from build123d import *

# Parameters (mm, degrees)
F3_START = -35.13478
F3_DEPTH = 29.12792
F4_SIZE  = 10.16
F5_R     = 93.5075941329
F6_DEPTH = 127


with BuildPart() as f1:
    # F0 (on Front) → F1 (revolve)
    with BuildSketch(Plane.XZ):
        Polygon((0, 127), (0, 0), (457.2, 0), (457.2, 38.1), (433.5165438938, 38.1), (433.5165438938, 106.68), (398.78, 106.68), (398.78, 152.4), (43.18, 152.4), (43.18, 127), align=None)
    revolve(axis=Axis((228.6, 0, 0), (1, 0, 0)))

    # F2 (on Top) → F3 (cut)
    with BuildSketch(Plane.XY.offset(F3_START)):
        with BuildLine():
            Line((435.6053211212, 11.4893475547), (390.5868865967, 11.4893475547))
            ThreePointArc((390.5868865967, 11.4893475547), (377.9254574746, -1.1720815673), (390.5868865967, -13.8335106894))
            Line((390.5868865967, -13.8335106894), (435.6053211212, -13.8335106894))
            ThreePointArc((435.6053211212, -13.8335106894), (448.2667502433, -1.1720815673), (435.6053211212, 11.4893475547))
        make_face()
    extrude(amount=-F3_DEPTH, mode=Mode.SUBTRACT)

    # F4
    f4_edges = [f1.edges().sort_by_distance(p)[0] for p in [
        (43.18, 0, -152.4),
        (398.78, 0, -152.4),
    ]]
    chamfer(f4_edges, length=F4_SIZE)

    # F5 (on face) → F6 (join)
    with BuildSketch(Plane(origin=(0, 0, 0), x_dir=(0, -1, 0), z_dir=(-1, 0, 0))):
        with Locations((-8.3505315706, -17.3037741333)):
            Circle(F5_R)
    extrude(amount=F6_DEPTH)


solid = f1.part
Can you work these out from the model? Positions are in its coordinate system, mm. A direction names the side the tool comes from. Coordinates: 2 decimals unless noted, no trailing zeros. Write each loop counter-clockwise with the first axis right and the second up, starting at its lowest first coordinate (ties: lowest second). Pieces come first, ordered by that corner, then holes. Notation, with made-up numbers: (28.5, 2) -> (64.5, 2) arc R16 cw to (64.5, 12) -> close; hole circle Ø1 at (80, 25.5). An arc over 180 degrees is marked (long way). Answer as CSV lines item,"result".
1) On a 3-axis mill with a long thin cutter (end or side, diameter ignored), from which of +Z, -Z, +X, -X, +Y, -Y can I reach the whole of each face in a straight line? I mean faces 1 (the cylindrical face through (445.19, -11.44, 36.34)), 2 (the cylindrical face through (21.29, 123.98, -27.53)), 3 (the cylindrical face through (448.264, -1.45, -36.274)). Say none if no direction works.
Check result:
face 1,"+X"
face 2,"-X"
face 3,"-Z"
2) If I drill on line 1 (X direction, y = -44.5, z = 92.5); line 2 (Y direction, x = 80, z = 2); line 3 (X direction, y = 18, z = -90.5), over which ranges is the centre line in solid material (lowest first)? Write a range as from..to.
Check result:
line 1,"0..433.52"
line 2,"-152.39..152.39"
line 3,"-127..433.52"
3) If we section it at B-B on y = 0: Please give me the cut outline in (x, z).
Check result:
outline,"(-127, -110.44) -> (0, -110.44) -> (0, -127) -> (43.18, -127) -> (43.18, -142.24) -> (53.34, -152.4) -> (388.62, -152.4) -> (398.78, -142.24) -> (398.78, -106.68) -> (433.52, -106.68) -> (433.52, -64.26) -> (377.98, -64.26) -> (377.98, -35.13) -> (448.21, -35.13) -> (448.21, -38.1) -> (457.2, -38.1) -> (457.2, 38.1) -> (433.52, 38.1) -> (433.52, 106.68) -> (398.78, 106.68) -> (398.78, 142.24) -> (388.62, 152.4) -> (53.34, 152.4) -> (43.18, 142.24) -> (43.18, 127) -> (0, 127) -> (0, 75.83) -> (-127, 75.83) -> close"
4) If we section it at A-A on z = 0: Please give me the cut outline in (x, y), then the cut area to 3 significant figures.
Check result:
outline,"(-127, -83.54) -> (0, -83.54) -> (0, -127) -> (43.18, -127) -> (43.18, -142.24) -> (53.34, -152.4) -> (388.62, -152.4) -> (398.78, -142.24) -> (398.78, -106.68) -> (433.52, -106.68) -> (433.52, -38.1) -> (457.2, -38.1) -> (457.2, 38.1) -> (433.52, 38.1) -> (433.52, 106.68) -> (398.78, 106.68) -> (398.78, 142.24) -> (388.62, 152.4) -> (53.34, 152.4) -> (43.18, 142.24) -> (43.18, 127) -> (0, 127) -> (0, 100.24) -> (-127, 100.24) -> close"
area,"152,000 mm²"
5) Will these pins go through, and if not, where does the flat tip stop? P1, Ø1.5, axis at y = -73, z = 119.5, coming from the -X side; P2, Ø2, axis at x = 342.5, y = 77, coming from the -Z side; P3, Ø1.5, axis at x = 319, y = -40.5, coming from the -Z side.
Check result:
P1,"x = 43.18"
P2,"z = -132.1"
P3,"z = -147.12"
6) If we section it at C-C on x = 116: Please give me the cut outline in (y, z), then the cut area to 3 significant figures.
Check result:
outline,"circle Ø304.8 at (0, 0)"
area,"73,000 mm²"
7) If we mould it in two halves opening along Z, with no side actions, what happens to faces 4 (the flat face through (-127, 10, -16)), 5 (the cylindrical face through (218.63, 92.73, -120.94)), 6 (the cylindrical face through (377.93, -0.89, -49.49))? For each: +Z half, -Z half, draft (parallel to the pull), parting line (faces both ways), or undercut.
Check result:
face 4,"draft"
face 5,"parting line"
face 6,"undercut"
